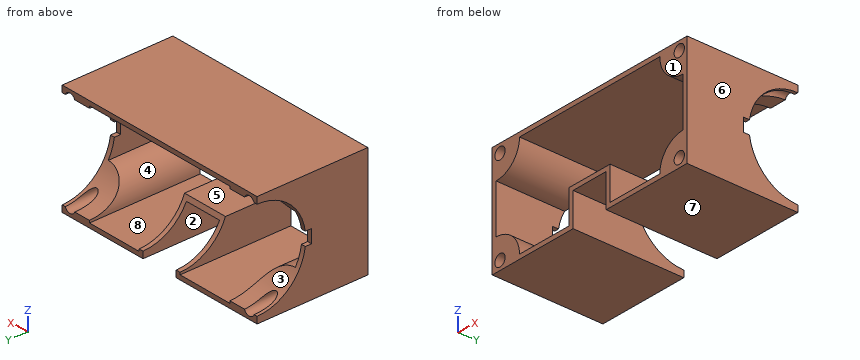
```python
from build123d import *

# Parameters (mm, degrees)
SKETCH1_R           = 1.325
BOSS_EXTRUDE1_DEPTH = 25
SKETCH3_R           = 11
CUT_EXTRUDE1_DEPTH  = 58.957500418
SKETCH4_W           = 3
SKETCH4_H           = 1.5
CUT_EXTRUDE2_DEPTH  = 58.957500548


with BuildPart() as part:
    # Sketch1 → Boss-Extrude1 (new body)
    with BuildSketch(Plane(origin=(0, 0, 0), x_dir=(1, 0, 0), z_dir=(0, 1, 0))):
        Polygon((-25, -9.700592993), (25, -9.700592993), (25, 15.299407007), (4.25, 15.299407007), (4.25, 7.799407007), (-4.25, 7.799407007), (-4.25, 15.299407007), (-25, 15.299407007), align=None)
        with Locations(Location((-23, 13.299407007, 0), (0, 0, 270))):
            Circle(SKETCH1_R, mode=Mode.SUBTRACT)
        with Locations(Location((23, 13.299407007, 0), (0, 0, 270))):
            Circle(SKETCH1_R, mode=Mode.SUBTRACT)
        with Locations(Location((23, -7.700592993, 0), (0, 0, 270))):
            Circle(SKETCH1_R, mode=Mode.SUBTRACT)
        with Locations(Location((-23, -7.700592993, 0), (0, 0, 270))):
            Circle(SKETCH1_R, mode=Mode.SUBTRACT)
        with BuildLine():
            Line((-5.25, 14.299407007), (-5.25, 6.799407007))
            Line((-5.25, 6.799407007), (5.25, 6.799407007))
            Line((5.25, 6.799407007), (5.25, 14.299407007))
            Line((5.25, 14.299407007), (18, 14.299407007))
            ThreePointArc((18, 14.299407007), (19.757359313, 10.05676632), (24, 8.299407007))
            Line((24, 8.299407007), (24, -2.700592993))
            ThreePointArc((24, -2.700592993), (19.757359313, -4.457952306), (18, -8.700592993))
            Line((18, -8.700592993), (-18, -8.700592993))
            ThreePointArc((-18, -8.700592993), (-19.757359313, -4.457952306), (-24, -2.700592993))
            Line((-24, -2.700592993), (-24, 8.299407007))
            ThreePointArc((-24, 8.299407007), (-19.757359313, 10.05676632), (-18, 14.299407007))
            Line((-18, 14.299407007), (-5.25, 14.299407007))
        make_face(mode=Mode.SUBTRACT)
    extrude(amount=BOSS_EXTRUDE1_DEPTH)

    # Sketch3 → Cut-Extrude1 (cut, through all)
    with BuildSketch(Plane(origin=(25, 0, 0), x_dir=(0, 0, -1), z_dir=(1, 0, 0))):
        with Locations((2.799407007, 25)):
            Circle(SKETCH3_R)
    extrude(amount=-CUT_EXTRUDE1_DEPTH, mode=Mode.SUBTRACT)

    # Sketch4 → Cut-Extrude2 (cut, through all)
    with BuildSketch(Plane(origin=(25, 0, 0), x_dir=(0, 0, -1), z_dir=(1, 0, 0))):
        with Locations((2.799407007, 13.45)):
            Rectangle(SKETCH4_W, SKETCH4_H)
    extrude(amount=-CUT_EXTRUDE2_DEPTH, mode=Mode.SUBTRACT)


solid = part.part
```
Geometry: final body of the model. Coordinates: model frame, mm. Face numbers are marked on the shaded views. A direction names the side the tool comes from. Coordinates: 2 decimals unless noted, no trailing zeros. Order: outer loops, then holes, each group sorted by start corner. A loop starts at its lowest first (then second) coordinate and runs counter-clockwise, first axis right, second up. Notation, with made-up numbers: (68, -4) -> (96, -4) arc R25 cw to (96, 12) -> close; hole circle Ø4 at (62, 4). An arc over 180 degrees is marked (long way). Use CSV: the item, a comma, the result in double quotes.
1) Access query for the marked faces 1, 2, 3 and 4. Directions: +Z, -Z, +X, -X, +Y, -Y. A direction counts if a zero-diameter tool reaches every point of the face in a straight line with its end or side. Return the directions, or none.
Findings:
face 1,"+Z, -Z, +X, -X, -Y"
face 2,"-Z, +Y, -Y"
face 3,"+X, -X, +Y"
face 4,"+Y, -Y"
2) Mould query, pull axis Z, two halves, no side actions, for the marked faces 5, 6, 7 and 8. Classes: +Z half, -Z half, draft (parallel to the pull), parting line (faces both ways), or undercut.
Findings:
face 5,"undercut"
face 6,"draft"
face 7,"-Z half"
face 8,"undercut"
3) Section B-B on y = 11. Output: boundary loops of the cut face in (x, z) (3 decimals), then the cut area to 3 significant figures.
Findings:
outline,"(-25, -15.299) -> (-4.25, -15.299) -> (-4.25, -7.799) -> (4.25, -7.799) -> (4.25, -15.299) -> (25, -15.299) -> (25, 9.701) -> (-25, 9.701) -> close; hole circle Ø2.65 at (-23, -13.299); hole circle Ø2.65 at (-23, 7.701); hole (-24, -8.299) arc R6 cw to (-18, -14.299) -> (-5.25, -14.299) -> (-5.25, -6.799) -> (5.25, -6.799) -> (5.25, -14.299) -> (18, -14.299) arc R6 cw to (24, -8.299) -> (24, 2.701) arc R6 cw to (18, 8.701) -> (-18, 8.701) arc R6 cw to (-24, 2.701) -> close; hole circle Ø2.65 at (23, -13.299); hole circle Ø2.65 at (23, 7.701)"
area,"252 mm^2"
4) Line query: line 1 (X direction, y = 14.5, z = -8); line 2 (X direction, y = 7.25, z = 1.75); line 3 (X direction, y = 5, z = 8.5). Output: solid intervals per line, ascending.
Findings:
line 1,"x = -25 to -24, -5.25 to -4.25, 4.25 to 5.25, 24 to 25"
line 2,"x = -25 to -24, 24 to 25"
line 3,"x = -25 to -24.06, -21.94 to -18, 18 to 21.94, 24.06 to 25"
5) Section A-A on x = 10. Output: boundary loops of the cut face in (y, z), then the cut area to 3 significant figures.
Findings:
outline,"(0, -15.3) -> (25, -15.3) -> (25, -14.3) -> (0, -14.3) -> close; (0, 8.7) -> (25, 8.7) -> (25, 9.7) -> (0, 9.7) -> close"
area,"50.0 mm^2"
6) Section D-D on x = -23. Output: boundary loops of the cut face in (y, z), then the cut area to 3 significant figures.
Findings:
outline,"(0, -15.3) -> (25, -15.3) -> (25, -14.62) -> (0, -14.62) -> close; (0, -11.97) -> (18.93, -11.97) arc R11 cw to (15.52, -8.38) -> (0, -8.38) -> close; (0, 2.78) -> (15.52, 2.78) arc R11 cw to (18.93, 6.38) -> (0, 6.38) -> close; (0, 9.03) -> (25, 9.03) -> (25, 9.7) -> (0, 9.7) -> close"
area,"156 mm^2"
7) Section C-C on z = 0. Output: boundary loops of the cut face in (x, y), then the cut area to 3 significant figures.
Findings:
outline,"(-25, 0) -> (-24, 0) -> (-24, 14.36) -> (-25, 14.36) -> close; (24, 0) -> (25, 0) -> (25, 14.36) -> (24, 14.36) -> close"
area,"28.7 mm^2"
8) Pin query (flat end, axial travel): pin 1 Ø10 at (x, z) = (6.5, -2.5) entering from +Y. Return the tip coordinate at first contact, or that it passes through.
Findings:
pin 1,"stops at y = 14.98"
